from build123d import *

# Parameters (mm, degrees)
F0_W     = 127
F0_H     = 101.6
F1_DEPTH = 20.32
F3_DEPTH = 25.4


with BuildPart() as f1:
    # F0 (on Front) → F1 (new body)
    with BuildSketch(Plane.XZ):
        Rectangle(F0_W, F0_H)
    extrude(amount=F1_DEPTH)

    # F2 (on face) → F3 (cut)
    with BuildSketch(Plane.XZ.offset(20.32)):
        Polygon((5.893087, 50.8), (-9.746261, 50.8), (-9.746261, 39.665014), (-19.265864, 39.665014), (-19.265864, 29.012125), (-8.612975, 29.012125), (-8.612975, 19.039206), (4.306488, 19.039206), (4.306488, 29.238781), (13.599434, 29.238781), (13.599434, 39.665014), (5.893087, 39.665014), align=None)
    extrude(amount=-F3_DEPTH, mode=Mode.SUBTRACT)


solid = f1.part
Check sheet for the modelled part. Datum: model origin and axes. Units: mm. A direction names the side the tool comes from. Round coordinates to 2 decimals unless told otherwise and drop trailing zeros. Loops run counter-clockwise (first coordinate to the right, second up) from the corner with the lowest first, then second, coordinate; pieces in that order, holes last.
1. Sectioned sample at B-B on y = -15.25. Record the boundary of the cut face in (x, z).
2. Sectioned sample at D-D on x = -4.5. Record the boundary of the cut face in (y, z), and give its area (3 significant figures).
3. Set-up check for faces 4 (the flat face through (-9.746, -10, 45)), 5 (the flat face through (-1, 0, 1)), 6 (the flat face through (-14, -10, 39.665)): record each of +Z, -Z, +X, -X, +Y, -Y from which the full face is reachable in a straight line by a thin tool's end or side.
4. Mould release check, pull along Z, two halves, no side actions. Record for faces 1 (the flat face through (-1, -20.32, 1)), 2 (the flat face through (-2, -10, 19.039)), 3 (the flat face through (-14, -10, 29.012)): released by +Z, released by -Z, zero draft, split by the parting line, or undercut.
5. Sectioned sample at C-C on z = 41. Record the boundary of the cut face in (x, y), and give its area (3 significant figures).
6. Sectioned sample at A-A on z = 26. Record the boundary of the cut face in (x, y).
7. Scan lines: probe 1 along X at (y, z) = (-0.75, 44.5); probe 2 along X at (y, z) = (-1.75, 36.5); probe 3 along Z at (x, y) = (7.5, -18). Record each from-to range of solid material in increasing order.
Recorded:
1. outline: (-63.5, -50.8) - (63.5, -50.8) - (63.5, 50.8) - (5.89, 50.8) - (5.89, 39.67) - (13.6, 39.67) - (13.6, 29.24) - (4.31, 29.24) - (4.31, 19.04) - (-8.61, 19.04) - (-8.61, 29.01) - (-19.27, 29.01) - (-19.27, 39.67) - (-9.75, 39.67) - (-9.75, 50.8) - (-63.5, 50.8) - close
2. outline: (-20.32, -50.8) - (0, -50.8) - (0, 19.04) - (-20.32, 19.04) - close
2. area: 1,420 mm2
3. face 4: +Z, +Y, -Y
3. face 5: +Z, -Z, +X, -X, +Y
3. face 6: +Y, -Y
4. face 1: zero draft
4. face 2: released by +Z
4. face 3: undercut
5. outline: (-63.5, -20.32) - (-9.75, -20.32) - (-9.75, 0) - (-63.5, 0) - close; (5.89, -20.32) - (63.5, -20.32) - (63.5, 0) - (5.89, 0) - close
5. area: 2,260 mm2
6. outline: (-63.5, -20.32) - (-8.61, -20.32) - (-8.61, 0) - (-63.5, 0) - close; (4.31, -20.32) - (63.5, -20.32) - (63.5, 0) - (4.31, 0) - close
7. probe 1: x = -63.5 to -9.75, 5.89 to 63.5
7. probe 2: x = -63.5 to -19.27, 13.6 to 63.5
7. probe 3: z = -50.8 to 29.24, 39.67 to 50.8
